from build123d import *

# Parameters (mm, degrees)
F1_DEPTH    = 9
F2_T2_ANGLE = 69.5952889026
F2_T4_ANGLE = 54.4883301746
F2_T6_ANGLE = 143.7551987737
F3_R        = 1


# Not quite as in the source:
# - a fillet or chamfer that OpenCascade refuses, or shapes differently, is made with other operations: its cross-section is extruded or revolved along the edge and cut away or added


with BuildPart() as f1:
    # F0 (on Front) → F1 (new body)
    with BuildSketch(Plane.XZ):
        with BuildLine():
            ThreePointArc((14.7663247772, 11.9293080643), (12.944509625, 17.3914763041), (13.0025018007, 23.1491606683))
            ThreePointArc((13.0025018007, 23.1491606683), (11.8204746449, 22.132281974), (10.26218878, 22.0777325565))
            ThreePointArc((10.26218878, 22.0777325565), (8.5829178564, 16.9649844736), (4.9823031081, 12.9655198559))
            ThreePointArc((4.9823031081, 12.9655198559), (4.6861100149, 11.4138618351), (4.9823031081, 9.8622038143))
            ThreePointArc((4.9823031081, 9.8622038143), (10.3556125988, 8.6176722475), (14.7663247772, 11.9293080643))
        make_face()
    extrude(amount=F1_DEPTH)

    # F2: fillet of radius 1 on 3 edges, made by hand

    # F2_s1 → F2_t2 (revolve, cut)
    with BuildSketch(Plane(origin=(-1.9409501927, 0, 23.5660641142), x_dir=(0, 1, 0), z_dir=(-0.0820841468, 0, 0.9966254025))):
        with BuildLine():
            ThreePointArc((-8, -12.2787262208), (-8.7071067812, -12.5716194396), (-9, -13.2787262208))
            Line((-9, -13.2787262208), (-9, -12.2787262208))
            Line((-9, -12.2787262208), (-8, -12.2787262208))
        make_face()
    revolve(axis=Axis((-2.70136938, -9, 23.5034344039), (0, 1, 0)), revolution_arc=F2_T2_ANGLE, mode=Mode.SUBTRACT)

    # F2_s3 → F2_t4 (revolve, cut)
    with BuildSketch(Plane(origin=(0.9320888174, 0, -1.2745523028), x_dir=(0, 1, 0), z_dir=(0.5902994367, 0, -0.8071843501))):
        with BuildLine():
            ThreePointArc((-8, 18.7819322745), (-8.7071067812, 18.4890390557), (-9, 17.7819322745))
            Line((-9, 17.7819322745), (-9, 18.7819322745))
            Line((-9, 18.7819322745), (-8, 18.7819322745))
        make_face()
    revolve(axis=Axis((30.156216129, -9, 20.0972519028), (0, 1, 0)), revolution_arc=F2_T4_ANGLE, mode=Mode.SUBTRACT)

    # F2_s5 → F2_t6 (revolve, cut)
    with BuildSketch(Plane(origin=(-4.2476398352, 0, 7.3417188573), x_dir=(0, 1, 0), z_dir=(-0.5007864485, 0, 0.8655708712))):
        with BuildLine():
            ThreePointArc((-8, -8.7783825872), (-8.7071067812, -9.071275806), (-9, -9.7783825872))
            Line((-9, -9.7783825872), (-9, -8.7783825872))
            Line((-9, -8.7783825872), (-8, -8.7783825872))
        make_face()
    revolve(axis=Axis((9.0052261238, -9, 15.0093240152), (0, -1, 0)), revolution_arc=F2_T6_ANGLE, mode=Mode.SUBTRACT)

    # F3#2 (call 1 of 2: OpenCascade refuses the feature's edges together)
    f3_2_edges = [f1.edges().sort_by_distance(p)[0] for p in [
        (8.582918, 0, 16.964984),
    ]]
    fillet(f3_2_edges, radius=F3_R)

    # F3 (call 2 of 2)
    f3_edges = [f1.edges().sort_by_distance(p)[0] for p in [
        (12.94451, 0, 17.391476),
        (10.355613, 0, 8.617672),
    ]]
    fillet(f3_edges, radius=F3_R)


solid = f1.part
Build history of the part. All positions in model axes, mm. Coordinates: 2 decimals unless noted, no trailing zeros. Order: outer loops, then holes, each group sorted by start corner. A loop starts at its lowest first (then second) coordinate and runs counter-clockwise, first axis right, second up. Notation, with made-up numbers: (-33, -26.75) -> (-25, -26.75) arc R18 ccw to (-25, 2.25) -> close; hole circle Ø2 at (-13.75, 63.5). An arc over 180 degrees is marked (long way). One line per item, written item: value.
(1) Mould opens along Z. For faces 1 (the cylindrical face through (8.62, -4.45, 17.03)), 2 (the cylindrical face through (10.278, -4.451, 8.602)), 3 (the flat face through (10, 0, 13)), 4 (the cylindrical face through (12.957, -4.451, 17.312)) say: pulls with the +Z half, pulls with the -Z half, needs draft (parallel to the pull), parting line crosses it, or undercut.
Checked values:
face 1: pulls with the +Z half
face 2: pulls with the -Z half
face 3: needs draft
face 4: undercut
(2) Probe line 1 (Y direction, x = 9.5, z = 16.75); line 2 (Z direction, x = 7.75, y = -5.5); line 3 (X direction, y = -8.25, z = 14.75). List the from-to ranges inside material, lowest first. Write a range as [from, to].
Checked values:
line 1: [-9, 0]
line 2: [8.6, 15.7]
line 3: [7.01, 13.54]
(3) Slice it at A-A, the plane y = -7.75. List the corners of the cut face in (x, z), plus the area to 3 significant figures.
Checked values:
outline: (4.98, 9.86) arc R6.53 ccw to (14.77, 11.93) arc R17.42 cw to (13, 23.15) arc R2.35 cw to (10.26, 22.08) arc R13.04 cw to (4.98, 12.97) arc R4.21 ccw to start
area: 79.5 mm2
(4) Drop flat-ended pins along their axis: pin 1 Ø3 at (y, z) = (-8, 15) entering from +X; pin 2 Ø2 at (y, z) = (-4.5, 19) entering from +X; pin 3 Ø1.5 at (y, z) = (-5, 15.5) entering from +X; pin 4 Ø3 at (x, z) = (10, 18.5) entering from -Y. Give the stop position or say it passes through.
Checked values:
pin 1: x = 14.03
pin 2: x = 12.86
pin 3: x = 13.57
pin 4: y = -9
